from build123d import *

# Parameters (mm, degrees)
SKETCH1_R                  = 6.5
SKETCH1_R_2                = 3
SKETCH1_R_3                = 4
BASE_FLANGE1_DEPTH         = 1
FILLET1_R                  = 5
SKETCHED_START             = 16.78876
SKETCHED_BEND1_OUTLINE_W   = 170
SKETCHED_BEND1_OUTLINE_H   = 1
SKETCHED_BEND1_DEPTH       = 13.21124
SKETCHED_START_2           = -30
SKETCHED_BEND1_2_OUTLINE_W = 170
SKETCHED_BEND1_2_OUTLINE_H = 1
SKETCHED_BEND1_2_DEPTH     = 13.18876
SKETCHED_START_3           = 16
SKETCHED_BEND1_3_DEPTH     = 0.0274
SKETCHED_START_4           = -16.01124
SKETCHED_BEND1_4_DEPTH     = 0.01124
SKETCHED_START_5           = -17
SKETCHED_BEND1_5_DEPTH     = 2
SKETCHED_START_6           = 15
SKETCHED_BEND1_6_DEPTH     = 2
SKETCHED_START_7           = -40.18
SKETCHED_BEND1_7_DEPTH     = 170
FILLET2_R                  = 1
F_6_CLEARANCE_HOLE2_D      = 3.7973
CUT_EXTRUDE1_DEPTH         = 10


with BuildPart() as part:
    # Base-Flange1: sheet metal written as solids
    # Sketch1 → Base-Flange1 (new body)
    with BuildSketch(Plane.XY):
        Polygon((-30, 129.82), (30, 129.82), (30, -40.18), (15, -40.18), (15, -75.18), (-15, -75.18), (-15, -40.18), (-30, -40.18), align=None)
        with Locations((0, -60.18)):
            Circle(SKETCH1_R, mode=Mode.SUBTRACT)
        with Locations((0, 114.82)):
            Circle(SKETCH1_R_2, mode=Mode.SUBTRACT)
        with Locations((0, 86.82)):
            Circle(SKETCH1_R_3, mode=Mode.SUBTRACT)
        Polygon((-26, 114.82), (-19, 108.82), (-19, 90.82), (-26, 84.82), align=None, mode=Mode.SUBTRACT)
        Polygon((-26, 78.82), (-19, 84.82), (-19, 54.82), (-26, 60.82), align=None, mode=Mode.SUBTRACT)
        Polygon((-26, 24.82), (-26, 54.82), (-19, 48.82), (-19, 30.82), align=None, mode=Mode.SUBTRACT)
        Polygon((19, 30.82), (26, 24.82), (26, 54.82), (19, 48.82), align=None, mode=Mode.SUBTRACT)
        Polygon((19, 54.82), (26, 60.82), (26, 78.82), (19, 84.82), align=None, mode=Mode.SUBTRACT)
        Polygon((19, 90.82), (26, 84.82), (26, 114.82), (19, 108.82), align=None, mode=Mode.SUBTRACT)
    extrude(amount=-BASE_FLANGE1_DEPTH)

    # Fillet1
    fillet1_edges = [part.edges().sort_by_distance(p)[0] for p in [
        (-30, 129.82, -0.5),
        (30, 129.82, -0.5),
        (30, -40.18, -0.5),
        (15, -75.18, -0.5),
        (-15, -75.18, -0.5),
        (-30, -40.18, -0.5),
    ]]
    fillet(fillet1_edges, radius=FILLET1_R)

    # Sketched Bend1: read off the stored shape, not the designer's step
    # Sketched Bend1 outline → Sketched Bend1 (cut)
    with BuildSketch(Plane.YZ.offset(SKETCHED_START)):
        with Locations((44.82, -0.5)):
            Rectangle(SKETCHED_BEND1_OUTLINE_W, SKETCHED_BEND1_OUTLINE_H)
    extrude(amount=SKETCHED_BEND1_DEPTH, mode=Mode.SUBTRACT)

    # Sketched Bend1 2 outline → Sketched Bend1 2 (cut)
    with BuildSketch(Plane.YZ.offset(SKETCHED_START_2)):
        with Locations((44.82, -0.5)):
            Rectangle(SKETCHED_BEND1_2_OUTLINE_W, SKETCHED_BEND1_2_OUTLINE_H)
    extrude(amount=SKETCHED_BEND1_2_DEPTH, mode=Mode.SUBTRACT)

    # Sketched Bend1 3 outline → Sketched Bend1 3 (add)
    with BuildSketch(Plane.YZ.offset(SKETCHED_START_3)):
        with BuildLine():
            Line((129.82, -9.64380551), (129.82, -1))
            Line((129.82, -1), (-40.18, -1))
            Line((-40.18, -1), (-40.18, -9.64380551))
            ThreePointArc((-40.18, -9.64380551), (-38.715533906, -13.179339416), (-35.18, -14.64380551))
            Line((-35.18, -14.64380551), (124.82, -14.64380551))
            ThreePointArc((124.82, -14.64380551), (128.355533906, -13.179339416), (129.82, -9.64380551))
        make_face()
        Polygon((30.82, -3.64380551), (48.82, -3.64380551), (54.82, -10.64380551), (24.82, -10.64380551), align=None, mode=Mode.SUBTRACT)
        Polygon((54.82, -3.64380551), (84.82, -3.64380551), (78.82, -10.64380551), (60.82, -10.64380551), align=None, mode=Mode.SUBTRACT)
        Polygon((90.82, -3.64380551), (108.82, -3.64380551), (114.82, -10.64380551), (84.82, -10.64380551), align=None, mode=Mode.SUBTRACT)
    extrude(amount=SKETCHED_BEND1_3_DEPTH)

    # Sketched Bend1 4 outline → Sketched Bend1 4 (add)
    with BuildSketch(Plane.YZ.offset(SKETCHED_START_4)):
        with BuildLine():
            Line((129.82, -9.64380551), (129.82, -1))
            Line((129.82, -1), (-40.18, -1))
            Line((-40.18, -1), (-40.18, -9.64380551))
            ThreePointArc((-40.18, -9.64380551), (-38.715533906, -13.179339416), (-35.18, -14.64380551))
            Line((-35.18, -14.64380551), (124.82, -14.64380551))
            ThreePointArc((124.82, -14.64380551), (128.355533906, -13.179339416), (129.82, -9.64380551))
        make_face()
        Polygon((30.82, -3.64380551), (48.82, -3.64380551), (54.82, -10.64380551), (24.82, -10.64380551), align=None, mode=Mode.SUBTRACT)
        Polygon((54.82, -3.64380551), (84.82, -3.64380551), (78.82, -10.64380551), (60.82, -10.64380551), align=None, mode=Mode.SUBTRACT)
        Polygon((90.82, -3.64380551), (108.82, -3.64380551), (114.82, -10.64380551), (84.82, -10.64380551), align=None, mode=Mode.SUBTRACT)
    extrude(amount=SKETCHED_BEND1_4_DEPTH)

    # Sketched Bend1 5 outline → Sketched Bend1 5 (add)
    with BuildSketch(Plane.YZ.offset(SKETCHED_START_5)):
        with BuildLine():
            Line((129.82, -9.64380551), (129.82, -1))
            Line((129.82, -1), (-40.18, -1))
            Line((-40.18, -1), (-40.18, -9.64380551))
            ThreePointArc((-40.18, -9.64380551), (-38.715533906, -13.179339416), (-35.18, -14.64380551))
            Line((-35.18, -14.64380551), (124.82, -14.64380551))
            ThreePointArc((124.82, -14.64380551), (128.355533906, -13.179339416), (129.82, -9.64380551))
        make_face()
        Polygon((30.82, -3.64380551), (48.82, -3.64380551), (54.82, -10.64380551), (24.82, -10.64380551), align=None, mode=Mode.SUBTRACT)
        Polygon((54.82, -3.64380551), (84.82, -3.64380551), (78.82, -10.64380551), (60.82, -10.64380551), align=None, mode=Mode.SUBTRACT)
        Polygon((90.82, -3.64380551), (108.82, -3.64380551), (114.82, -10.64380551), (84.82, -10.64380551), align=None, mode=Mode.SUBTRACT)
    extrude(amount=SKETCHED_BEND1_5_DEPTH)

    # Sketched Bend1 6 outline → Sketched Bend1 6 (add)
    with BuildSketch(Plane.YZ.offset(SKETCHED_START_6)):
        with BuildLine():
            Line((129.82, -9.64380551), (129.82, -1))
            Line((129.82, -1), (-40.18, -1))
            Line((-40.18, -1), (-40.18, -9.64380551))
            ThreePointArc((-40.18, -9.64380551), (-38.715533906, -13.179339416), (-35.18, -14.64380551))
            Line((-35.18, -14.64380551), (124.82, -14.64380551))
            ThreePointArc((124.82, -14.64380551), (128.355533906, -13.179339416), (129.82, -9.64380551))
        make_face()
        Polygon((30.82, -3.64380551), (48.82, -3.64380551), (54.82, -10.64380551), (24.82, -10.64380551), align=None, mode=Mode.SUBTRACT)
        Polygon((54.82, -3.64380551), (84.82, -3.64380551), (78.82, -10.64380551), (60.82, -10.64380551), align=None, mode=Mode.SUBTRACT)
        Polygon((90.82, -3.64380551), (108.82, -3.64380551), (114.82, -10.64380551), (84.82, -10.64380551), align=None, mode=Mode.SUBTRACT)
    extrude(amount=SKETCHED_BEND1_6_DEPTH)

    # Sketched Bend1 7 outline → Sketched Bend1 7 (cut)
    with BuildSketch(Plane(origin=(0, 0, 0), x_dir=(1, 0, 0), z_dir=(0, 1, 0)).offset(SKETCHED_START_7)):
        with BuildLine():
            ThreePointArc((-16, 2), (-15.707106781, 1.292893219), (-15, 1))
            Line((-15, 1), (-15, 14.64380551))
            Line((-15, 14.64380551), (-16, 14.64380551))
            Line((-16, 14.64380551), (-16, 2))
        make_face()
        with BuildLine():
            ThreePointArc((17, 2), (16.414213562, 0.585786438), (15, 0))
            Line((15, 0), (16.78876, 0))
            Line((16.78876, 0), (16.78876, 1))
            Line((16.78876, 1), (17, 1))
            Line((17, 1), (17, 2))
        make_face()
        with BuildLine():
            ThreePointArc((-15, 0), (-16.414213562, 0.585786438), (-17, 2))
            Line((-17, 2), (-17, 1))
            Line((-17, 1), (-16.81124, 1))
            Line((-16.81124, 1), (-16.81124, 0))
            Line((-16.81124, 0), (-15, 0))
        make_face()
        with BuildLine():
            ThreePointArc((15, 1), (15.707106781, 1.292893219), (16, 2))
            Line((16, 2), (16, 14.64380551))
            Line((16, 14.64380551), (15, 14.64380551))
            Line((15, 14.64380551), (15, 1))
        make_face()
    extrude(amount=SKETCHED_BEND1_7_DEPTH, mode=Mode.SUBTRACT)

    # Fillet2
    fillet2_edges = [part.edges().sort_by_distance(p)[0] for p in [
        (-16.5, 90.82, -3.64380551),
        (-16.5, 84.82, -10.64380551),
        (-16.5, 114.82, -10.64380551),
        (-16.5, 108.82, -3.64380551),
        (-16.5, 84.82, -3.64380551),
        (-16.5, 54.82, -3.64380551),
        (-16.5, 60.82, -10.64380551),
        (-16.5, 78.82, -10.64380551),
        (-16.5, 24.82, -10.64380551),
        (-16.5, 54.82, -10.64380551),
        (-16.5, 48.82, -3.64380551),
        (-16.5, 30.82, -3.64380551),
        (16.5, 24.82, -10.64380551),
        (16.5, 30.82, -3.64380551),
        (16.5, 48.82, -3.64380551),
        (16.5, 54.82, -10.64380551),
        (16.5, 60.82, -10.64380551),
        (16.5, 54.82, -3.64380551),
        (16.5, 84.82, -3.64380551),
        (16.5, 78.82, -10.64380551),
        (16.5, 84.82, -10.64380551),
        (16.5, 90.82, -3.64380551),
        (16.5, 108.82, -3.64380551),
        (16.5, 114.82, -10.64380551),
    ]]
    fillet(fillet2_edges, radius=FILLET2_R)

    # #6 Clearance Hole2 (through all)
    with Locations(Plane.XY):
        with Locations((-8, 67), (8, 67), (0, 17), (-8, -33), (8, -33), (-10, -49.375603427), (10, -49.375603427), (-10, -69.375603427), (10, -69.375603427), (28.213155681, -64.18604224)):
            Hole(F_6_CLEARANCE_HOLE2_D / 2)

    # Sketch13 → Cut-Extrude1 (cut)
    with BuildSketch(Plane.XY):
        with BuildLine():
            Line((-7.5, 3), (7.5, 3))
            ThreePointArc((7.5, 3), (10.5, 0), (7.5, -3))
            Line((7.5, -3), (-7.5, -3))
            ThreePointArc((-7.5, -3), (-10.5, 0), (-7.5, 3))
        make_face()
        with BuildLine():
            Line((-7.5, -17), (7.5, -17))
            ThreePointArc((7.5, -17), (10.5, -20), (7.5, -23))
            Line((7.5, -23), (-7.5, -23))
            ThreePointArc((-7.5, -23), (-10.5, -20), (-7.5, -17))
        make_face()
        with BuildLine():
            Line((-7.5, 28), (7.5, 28))
            ThreePointArc((7.5, 28), (10.5, 25), (7.5, 22))
            Line((7.5, 22), (-7.5, 22))
            ThreePointArc((-7.5, 22), (-10.5, 25), (-7.5, 28))
        make_face()
        with BuildLine():
            Line((-7.5, 48), (7.5, 48))
            ThreePointArc((7.5, 48), (10.5, 45), (7.5, 42))
            Line((7.5, 42), (-7.5, 42))
            ThreePointArc((-7.5, 42), (-10.5, 45), (-7.5, 48))
        make_face()
        with BuildLine():
            Line((-7.5, 68), (7.5, 68))
            ThreePointArc((7.5, 68), (10.5, 65), (7.5, 62))
            Line((7.5, 62), (-7.5, 62))
            ThreePointArc((-7.5, 62), (-10.5, 65), (-7.5, 68))
        make_face()
    extrude(amount=-CUT_EXTRUDE1_DEPTH, mode=Mode.SUBTRACT)


solid = part.part
Design review of the part built by this model. Coordinates are the model's own, in mm. A direction names the side the tool comes from. Round coordinates to 2 decimals unless told otherwise and drop trailing zeros. Write each loop counter-clockwise with the first axis right and the second up, starting at its lowest first coordinate (ties: lowest second). Pieces come first, ordered by that corner, then holes. Notation, with made-up numbers: (86.25, -33) - (142.25, -33) arc R13 cw to (142.25, -17) - close; hole circle Ø6 at (89.25, 54). An arc over 180 degrees is marked (long way). Return JSON: item names as keys, results as strings. Group by question number.
Item 1: Insertion check: P1, Ø1.1, axis at x = -16.5, y = 97.5, coming from the +Z side; P2, Ø3, axis at x = 4, y = 28, coming from the -Z side. Each pin has a flat end and moves straight along its axis. Give the tip position at first contact, or say it passes through.
Item 2: Machinability: for faces 4 (the face through (-16, 44, -11)), 5 (the face through (-16.51, 81.29, -7.76)), 6 (the face through (11.507, -70.531, -0.507)), which of the approach directions +Z, -Z, +X, -X, +Y, -Y give a long, thin tool a straight path to every point of the face, cutting with its end or side? Answer none if there is none.
Item 3: We need section C-C on x = 0. Give the number of separate pieces and of enclosed holes in the cut face, and give its area (3 significant figures).
Item 4: The part is to be moulded in two halves that separate along Y. For faces 1 (the face through (16, 44, -11)), 2 (the face through (16.493, 128.316, -13.218)), 3 (the face through (-0.521, 90.786, -0.493)), say which applies: pulls with the +Y half, pulls with the -Y half, needs draft (parallel to the pull), parting line crosses it, or undercut.
Item 5: For probe 1 along X at (y, z) = (23.5, -3.5); probe 2 along Z at (x, y) = (-14, -42.5); probe 3 along X at (y, z) = (71, -1.25), list the stretches that pass through material, from the lowest coordinate up. Write a range as [from, to].
Item 6: We need section A-A on y = 45. Write out the cut boundary in (x, z), and give its area (3 significant figures).
Item 7: We need section D-D on y = -60.18. Write out the cut boundary in (x, z).
Item 8: We need section B-B on y = 0. Write out the cut boundary in (x, z), and give its area (3 significant figures).
Model answer:
{
 "1": {"P1": "stops at z = -0.24", "P2": "stops at z = -1"},
 "2": {"face 4": "-Z, +Y, -Y", "face 5": "+X, -X", "face 6": "+Z, -Z"},
 "3": {"separate pieces": "10", "enclosed holes": "0", "area": "144 mm²"},
 "4": {"face 1": "needs draft", "face 2": "pulls with the +Y half", "face 3": "undercut"},
 "5": {"probe 1": "x = [-17, -16], [16, 17]", "probe 2": "z = [-1, 0]", "probe 3": "x = [-16.85, -15.66], [15.66, 16.85]"},
 "6": {"outline": "(-17, -14.64) - (-16, -14.64) - (-16, -10.64) - (-17, -10.64) - close; (-17, -3.64) - (-16, -3.64) - (-16, -2) arc R1 cw to (-15, -1) - (-10.5, -1) - (-10.5, 0) - (-15, 0) arc R2 ccw to (-17, -2) - close; (10.5, -1) - (15, -1) arc R1 cw to (16, -2) - (16, -3.64) - (17, -3.64) - (17, -2) arc R2 ccw to (15, 0) - (10.5, 0) - close; (16, -14.64) - (17, -14.64) - (17, -10.64) - (16, -10.64) - close", "area": "25.0 mm²"},
 "7": {"outline": "(-15, -1) - (-6.5, -1) - (-6.5, 0) - (-15, 0) - close; (6.5, -1) - (15, -1) - (15, 0) - (6.5, 0) - close"},
 "8": {"outline": "(-17, -14.64) - (-16, -14.64) - (-16, -2) arc R1 cw to (-15, -1) - (-10.5, -1) - (-10.5, 0) - (-15, 0) arc R2 ccw to (-17, -2) - close; (10.5, -1) - (15, -1) arc R1 cw to (16, -2) - (16, -14.64) - (17, -14.64) - (17, -2) arc R2 ccw to (15, 0) - (10.5, 0) - close", "area": "39.0 mm²"}
}
